```python
from build123d import *

# Parameters (mm, degrees)
EXTRUDE_1_DEPTH     = 300
CUT_EXTRUDE_1_DEPTH = 10


with BuildPart() as part:
    # Эскиз1 → Бобышка-Вытянуть1 (new body)
    with BuildSketch(Plane(origin=(0, 0, 0), x_dir=(0, 0, -1), z_dir=(1, 0, 0))):
        with BuildLine():
            Line((0, 7.524096324), (0, 6))
            Line((0, 6), (4.2, 6))
            ThreePointArc((4.2, 6), (4.765685425, 5.765685425), (5, 5.2))
            Line((5, 5.2), (5, 0.8))
            ThreePointArc((5, 0.8), (5.234314575, 0.234314575), (5.8, 0))
            Line((5.8, 0), (29.2, 0))
            ThreePointArc((29.2, 0), (29.765685425, 0.234314575), (30, 0.8))
            Line((30, 0.8), (30, 5.2))
            ThreePointArc((30, 5.2), (30.234314575, 5.765685425), (30.8, 6))
            Line((30.8, 6), (35, 6))
            Line((35, 6), (35, 7.5))
            Line((35, 7.5), (29.3, 7.5))
            ThreePointArc((29.3, 7.5), (28.734314575, 7.265685425), (28.5, 6.7))
            Line((28.5, 6.7), (28.5, 2.3))
            ThreePointArc((28.5, 2.3), (28.265685425, 1.734314575), (27.7, 1.5))
            Line((27.7, 1.5), (7.3, 1.5))
            ThreePointArc((7.3, 1.5), (6.734314575, 1.734314575), (6.5, 2.3))
            Line((6.5, 2.3), (6.5, 6.724096324))
            ThreePointArc((6.5, 6.724096324), (6.265685425, 7.289781749), (5.7, 7.524096324))
            Line((5.7, 7.524096324), (0, 7.524096324))
        make_face()
    extrude(amount=EXTRUDE_1_DEPTH)

    # Эскиз2 → Вырез-Вытянуть1 (cut)
    with BuildSketch(Plane(origin=(0, 1.5, 0), x_dir=(1, 0, 0), z_dir=(0, 1, 0))):
        with BuildLine():
            Line((57.050825201, 20.5), (95.873378283, 20.5))
            ThreePointArc((95.873378283, 20.5), (96.439063708, 20.265685425), (96.673378283, 19.7))
            Line((96.673378283, 19.7), (96.673378283, 16.3))
            ThreePointArc((96.673378283, 16.3), (96.439063708, 15.734314575), (95.873378283, 15.5))
            Line((95.873378283, 15.5), (57.050825201, 15.5))
            ThreePointArc((57.050825201, 15.5), (56.485139776, 15.734314575), (56.250825201, 16.3))
            Line((56.250825201, 16.3), (56.250825201, 19.7))
            ThreePointArc((56.250825201, 19.7), (56.485139776, 20.265685425), (57.050825201, 20.5))
        make_face()
        with BuildLine():
            Line((7.050825201, 20.5), (45.873378283, 20.5))
            ThreePointArc((45.873378283, 20.5), (46.439063708, 20.265685425), (46.673378283, 19.7))
            Line((46.673378283, 19.7), (46.673378283, 16.3))
            ThreePointArc((46.673378283, 16.3), (46.439063708, 15.734314575), (45.873378283, 15.5))
            Line((45.873378283, 15.5), (7.050825201, 15.5))
            ThreePointArc((7.050825201, 15.5), (6.485139776, 15.734314575), (6.250825201, 16.3))
            Line((6.250825201, 16.3), (6.250825201, 19.7))
            ThreePointArc((6.250825201, 19.7), (6.485139776, 20.265685425), (7.050825201, 20.5))
        make_face()
        with BuildLine():
            Line((107.050825201, 20.5), (145.873378283, 20.5))
            ThreePointArc((145.873378283, 20.5), (146.439063708, 20.265685425), (146.673378283, 19.7))
            Line((146.673378283, 19.7), (146.673378283, 16.3))
            ThreePointArc((146.673378283, 16.3), (146.439063708, 15.734314575), (145.873378283, 15.5))
            Line((145.873378283, 15.5), (107.050825201, 15.5))
            ThreePointArc((107.050825201, 15.5), (106.485139776, 15.734314575), (106.250825201, 16.3))
            Line((106.250825201, 16.3), (106.250825201, 19.7))
            ThreePointArc((106.250825201, 19.7), (106.485139776, 20.265685425), (107.050825201, 20.5))
        make_face()
        with BuildLine():
            Line((157.050825201, 20.5), (195.873378283, 20.5))
            ThreePointArc((195.873378283, 20.5), (196.439063708, 20.265685425), (196.673378283, 19.7))
            Line((196.673378283, 19.7), (196.673378283, 16.3))
            ThreePointArc((196.673378283, 16.3), (196.439063708, 15.734314575), (195.873378283, 15.5))
            Line((195.873378283, 15.5), (157.050825201, 15.5))
            ThreePointArc((157.050825201, 15.5), (156.485139776, 15.734314575), (156.250825201, 16.3))
            Line((156.250825201, 16.3), (156.250825201, 19.7))
            ThreePointArc((156.250825201, 19.7), (156.485139776, 20.265685425), (157.050825201, 20.5))
        make_face()
    extrude(amount=-CUT_EXTRUDE_1_DEPTH, mode=Mode.SUBTRACT)


solid = part.part
```
Geometry: final body of the model. Coordinates: model frame, mm. A direction names the side the tool comes from. Give positions to 0.01 mm unless a question says otherwise; leave off trailing zeros. Loops run counter-clockwise (first coordinate to the right, second up) from the corner with the lowest first, then second, coordinate; pieces in that order, holes last. Notation, with made-up numbers: (4, 3.25) - (55, 3.25) arc R27 cw to (55, 33.25) - close; hole circle Ø2 at (-22, 87.25). An arc over 180 degrees is marked (long way). Answer as CSV lines item,"result". Start each with the question number.
(1) Section query B-B (x = 248.5). Output: boundary loops of the cut face in (y, z).
(2) Reachability of faces 1 (the face through (148, 1.5, -18)), 2 (the face through (148, 7.5, -32)) from +Z, -Z, +X, -X, +Y, -Y: full face, straight path, thin tool, end or side. Return the list, or none.
(3) Pin query (flat end, axial travel): P1, Ø4, axis at x = 246.5, y = 2, coming from the +Z side; P2, Ø2, axis at x = 197.5, z = -2, coming from the -Y side; P3, Ø1.6, axis at x = 131, y = 1, coming from the -Z side. Return the tip coordinate at first contact, or that it passes through.
(4) Section query A-A (x = 37). Output: boundary loops of the cut face in (y, z).
(5) Ray query, line 1 along Z through (x, y) = (15, 4.25); line 2 along Z through (x, y) = (175.5, 6.75); line 3 along X through (y, z) = (0.5, -19). Return the intervals inside material, ascending. Write a range as [from, to].
(6) Section query C-C (z = -24). Output: boundary loops of the cut face in (x, y), and give its area (3 significant figures).
Worked answers:
1,outline,"(0, -29.2) arc R0.8 ccw to (0.8, -30) - (5.2, -30) arc R0.8 cw to (6, -30.8) - (6, -35) - (7.5, -35) - (7.5, -29.3) arc R0.8 ccw to (6.7, -28.5) - (2.3, -28.5) arc R0.8 cw to (1.5, -27.7) - (1.5, -7.3) arc R0.8 cw to (2.3, -6.5) - (6.72, -6.5) arc R0.8 ccw to (7.52, -5.7) - (7.52, 0) - (6, 0) - (6, -4.2) arc R0.8 cw to (5.2, -5) - (0.8, -5) arc R0.8 ccw to (0, -5.8) - close"
2,face 1,"+X, -X, +Y"
2,face 2,"+Z, -Z, +X, -X, +Y"
3,P1,"stops at z = -5"
3,P2,"stops at y = 6"
3,P3,"stops at z = -30"
4,outline,"(0, -29.2) arc R0.8 ccw to (0.8, -30) - (5.2, -30) arc R0.8 cw to (6, -30.8) - (6, -35) - (7.5, -35) - (7.5, -29.3) arc R0.8 ccw to (6.7, -28.5) - (2.3, -28.5) arc R0.8 cw to (1.5, -27.7) - (1.5, -20.5) - (0, -20.5) - close; (0, -15.5) - (1.5, -15.5) - (1.5, -7.3) arc R0.8 cw to (2.3, -6.5) - (6.72, -6.5) arc R0.8 ccw to (7.52, -5.7) - (7.52, 0) - (6, 0) - (6, -4.2) arc R0.8 cw to (5.2, -5) - (0.8, -5) arc R0.8 ccw to (0, -5.8) - close"
5,line 1,"z = [-30, -28.5], [-6.5, -5]"
5,line 2,"z = [-35, -28.5], [-6.5, 0]"
5,line 3,"x = [0, 6.25], [46.67, 56.25], [96.67, 106.25], [146.67, 156.25], [196.67, 300]"
6,outline,"(0, 0) - (300, 0) - (300, 1.5) - (0, 1.5) - close"
6,area,"450 mm^2"
